Autodesk Inventor part; units mm, degrees
ref_plane "Work Plane1" through (0, 0, -22) normal (0, 0, -1) x (-1, 0, 0)
ref_plane "YZ Plane" through (0, 0, 0) normal (1, 0, 0) x (0, 1, 0)
ref_plane "XZ Plane" through (0, 0, 0) normal (0, 1, 0) x (-1, 0, 0)
sketch "Sketch1" plane through (0, 0, 0) normal (0, 0, 1) x (1, 0, 0)
  line L0 (-2.3383, -4.05) -> (-4.6765, 0)
  line L1 (-4.6765, 0) -> (-2.3383, 4.05)
  line L2 (-2.3383, 4.05) -> (2.3383, 4.05)
  line L3 (2.3383, 4.05) -> (4.6765, 0)
  line L4 (4.6765, 0) -> (2.3383, -4.05)
  line L5 (2.3383, -4.05) -> (-2.3383, -4.05)
  point P0 (0, 0)
  point P1 (0, 0)
  dimension "d0" = 4.05
extrude "Extrusion1" add sketch "Sketch1" against normal blind 44
sketch "Sketch2" plane through (4.6765, 0, 0) normal (0.866, 0.5, 0) x (0, 0, -1)
  line L0 (0, 4.6765) -> (0, 0)
  line L1 (4.75, 5.1383) -> (7.25, 5.1383)
  line L2 (7.25, 5.1383) -> (7.25, -0.4617)
  line L3 (7.25, -0.4617) -> (4.75, -0.4617)
  line L4 (4.75, -0.4617) -> (4.75, 5.1383)
  line L5 (4.75, 5.1383) -> (7.25, -0.4617) construction
  line L6 (7.25, 5.1383) -> (4.75, -0.4617) construction
  point P0 (0, 2.3383)
  point P1 (6, 2.3383)
  dimension "d3" = 2.5
  dimension "d4" = 5.6
  dimension "d10" = 0
  dimension "d11" = 6
extrude "Extrusion2" [suppressed]
sketch "Sketch3" plane through (0, 0, 0) normal (0, 0, 1) x (1, 0, 0)
  circle A0 centre (0, 0) radius 1.5
  dimension "d7" = 3
extrude "Extrusion3" cut sketch "Sketch3" against normal blind 8
ref_plane "Work Plane1" through (0, 0, -22) normal (0, 0, -1) x (-1, 0, 0)
mirror "Mirror1" [suppressed]
sketch "Sketch4" plane through (1.5014, 4.1, -7.25) normal (0, 0, 1) x (1, 0, 0)
  line L0 (0, 0) -> (-4.5469, -2.6251)
  line L1 (-1.7469, -7.4749) -> (-4.5469, -2.6251)
  line L2 (2.8, -4.8497) -> (-1.7469, -7.4749)
  line L3 (-4.5469, -2.6251) -> (-4.5469, -5.8583)
  line L4 (-1.7469, -7.4749) -> (-4.5469, -5.8583)
  line L5 (-1.7469, -7.4749) -> (-4.5469, -2.6251)
  point P0 (-1.5014, -4.1)
  dimension "d12" = 120
  dimension "d13" = 120
extrude "Extrusion4" [suppressed]
sketch "Sketch5" plane through (-4.6765, 0, -44) normal (-0.866, -0.5, 0) x (0, 0, 1)
  line L0 (0, -4.6765) -> (0, 0)
  line L1 (4.75, 0.5197) -> (7.25, 0.5197)
  line L2 (7.25, 0.5197) -> (7.25, -5.0803)
  line L3 (7.25, -5.0803) -> (4.75, -5.0803)
  line L4 (4.75, -5.0803) -> (4.75, 0.5197)
  line L5 (4.75, 0.5197) -> (7.25, -5.0803) construction
  line L6 (7.25, 0.5197) -> (4.75, -5.0803) construction
  line L7 (0, -3.8671) -> (0, -0.8671)
  line L8 (0, -4.6765) -> (0, 0)
  line L9 (0, 0) -> (0, 2.3383)
  line L10 (0, 2.3383) -> (0, 0)
  line L11 (0, 0) -> (0, -4.6765)
  line L12 (0, -4.6765) -> (0, -7.0148)
  line L13 (0, -7.0148) -> (0, -4.6765)
  line L14 (9.5, -0.8671) -> (9.5, -3.8671)
  line L15 (0, -3.8671) -> (0, -0.8671)
  line L16 (44, -7.0148) -> (0, -7.0148)
  line L17 (44, 2.3383) -> (0, 2.3383)
  point P0 (44, -2.3383)
  point P1 (6, -2.2803)
  dimension "d16" = 2.5
  dimension "d17" = 5.6
  dimension "d18" = 6
  dimension "d25" = 1.9345
extrude "Extrusion5" [suppressed]
sketch "Sketch6" plane through (-1.5019, -4.1, -42.75) normal (0, 0, -1) x (-1, 0, 0)
  line L0 (-1.7472, 7.4751) -> (-4.5472, 2.6253)
  line L1 (-4.5472, 2.6253) -> (-4.5472, 5.8585)
  line L2 (-1.7472, 7.4751) -> (-4.5472, 5.8585)
  line L3 (2.7993, 4.8501) -> (-1.7472, 7.4751)
  line L4 (0, 0) -> (-4.5472, 2.6253)
  line L5 (-1.7472, 7.4751) -> (-4.5472, 2.6253)
  point P0 (-1.5019, 4.1)
  dimension "d21" = 120
  dimension "d22" = 120
extrude "Extrusion6" [suppressed]
sketch "Sketch8" plane through (0, 0, -44) normal (0, 0, -1) x (-1, 0, 0)
  line L0 (-2.8, 1.25) -> (2.8, 1.25)
  line L1 (2.8, 1.25) -> (2.8, -1.25)
  line L2 (2.8, -1.25) -> (-2.8, -1.25)
  line L3 (-2.8, -1.25) -> (-2.8, 1.25)
  circle A0 centre (0, 0) radius 1.5
  line L4 (-2.8, 1.25) -> (2.8, -1.25) construction
  line L5 (2.8, 1.25) -> (-2.8, -1.25) construction
  dimension "d32" = 5.6
  dimension "d33" = 2.5
extrude "Extrusion8" cut sketch "Sketch8" against normal blind 6.5 contours L0 A0 L2 L3 | L0 A0 L2 | L0 L1 L2 A0
sketch "Sketch9" plane through (-2.3383, 4.05, 0) normal (0, 1, 0) x (1, 0, 0)
  line L0 (4.6765, 0) -> (4.6765, 44)
  line L1 (0, 44) -> (4.6765, 44)
  line L2 (0, 0) -> (0, 44)
  line L3 (0, 0) -> (4.6765, 0)
  line L4 (5.1383, 44) -> (-0.4617, 44)
  line L5 (2.3383, 44) -> (2.3383, 0) construction
  line L6 (2.3383, 44) -> (46.3383, 44) construction
  circle A0 centre (2.3383, 39.5) radius 1.5
  dimension "d36" = 90
  dimension "d37" = 3
  dimension "d38" = 0
  dimension "d39" = 4.5
extrude "Extrusion9" cut sketch "Sketch9" against normal up to surface (8.1 mm away) contours A0
sketch "Sketch10" plane through (-2.8, 1.25, -44) normal (0, -1, 0) x (1, 0, 0)
  circle A0 centre (2.8, 4.5) radius 1.5
  line L0 (5.6, 0) -> (0, 0)
  line L1 (5.6, 0) -> (5.6, 6.5)
  line L2 (5.6, 6.5) -> (0, 6.5)
  line L3 (0, 0) -> (0, 6.5)
  line L4 (0, 6.5) -> (2.8, 8.1166)
  line L5 (0, 6.5) -> (3.9156, 6.5) construction
  line L6 (5.6, 6.5) -> (2.8, 8.1166)
  line L7 (5.6, 6.5) -> (8.8332, 6.5) construction
  line L8 (5.6, 6.5) -> (0, 6.5)
  point P0 (2.8, 44)
  dimension "d42" = 30
  dimension "d43" = 150
extrude "Extrusion10" cut sketch "Sketch10" along normal blind 2.5 contours L2 L4 L6
sketch "Sketch11" plane through (-2.3383, 4.05, 0) normal (0, 1, 0) x (1, 0, 0)
  circle A0 centre (2.3383, 39.5) radius 1.5
  line L0 (0, 0) -> (4.6765, 0)
  line L1 (4.6765, 0) -> (4.6765, 44)
  line L2 (0, 44) -> (4.6765, 44)
  line L3 (0, 0) -> (0, 44)
  line L4 (-0.4617, 0.8) -> (5.1383, 0.8)
  line L5 (5.1383, 0.8) -> (5.1383, 3.3)
  line L6 (5.1383, 3.3) -> (-0.4617, 3.3)
  line L7 (-0.4617, 3.3) -> (-0.4617, 0.8)
  line L8 (-0.4617, 0.8) -> (5.1383, 3.3) construction
  line L9 (5.1383, 0.8) -> (-0.4617, 3.3) construction
  point P0 (2.3383, 0)
  point P1 (2.3383, 2.05)
  dimension "d46" = 5.6
  dimension "d47" = 2.5
  dimension "d48" = 2.05
extrude "Extrusion11" cut sketch "Sketch11" against normal blind 5.85 contours L4 L7 L6 L3 | L3 L6 L1 L4 | L1 L6 L5 L4
sketch "Sketch12" plane through (2.3383, 4.05, -0.8) normal (0, 0, -1) x (-1, 0, 0)
  line L0 (5.1383, -0.7997) -> (4.6765, 0)
  line L1 (5.1383, -0.7997) -> (5.1383, -5.85)
  line L2 (5.1383, -5.85) -> (-0.4617, -5.85)
  line L3 (-0.4617, -0.7997) -> (-0.4617, -5.85)
  line L4 (0, 0) -> (-0.4617, -0.7997)
  line L5 (4.6765, 0) -> (0, 0)
  circle A0 centre (2.3383, -4.05) radius 1.5
  line L6 (5.1383, -5.85) -> (2.3383, -7.4666)
  line L7 (5.1383, -5.85) -> (8.4476, -5.85) construction
  line L8 (-0.4617, -5.85) -> (2.3383, -7.4666)
  line L9 (-0.4617, -5.85) -> (2.7714, -5.85) construction
  dimension "d52" = 150
  dimension "d53" = 30
extrude "Extrusion12" cut sketch "Sketch12" along normal up to surface (2.5 mm away) contours L6 L8 L2
properties part number "SupportSecondToCoverNew" material "ABS Plastic"
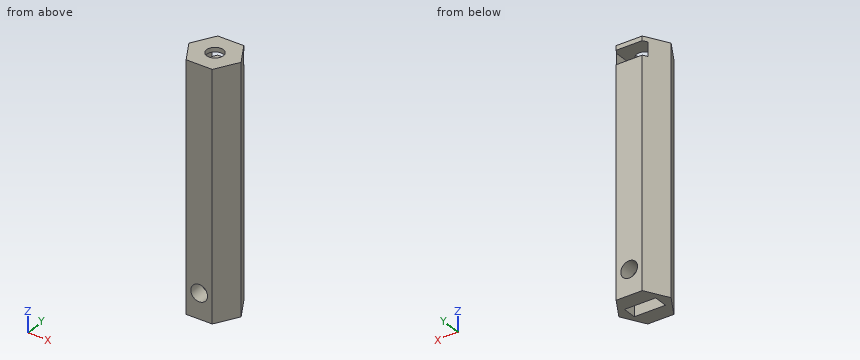
Part model, mm, in its own coordinate system. Round coordinates to 2 decimals unless told otherwise and drop trailing zeros. Loops run counter-clockwise (first coordinate to the right, second up) from the corner with the lowest first, then second, coordinate; pieces in that order, holes last. Notation, with made-up numbers: (9.5, 52) -> (32.5, 52) arc R20 ccw to (32.5, 61) -> close; hole circle Ø11 at (-6.75, -27.75). An arc over 180 degrees is marked (long way). Use CSV: the item, a comma, the result in double quotes. Start each with the question number.
1) Cut at D-D, the plane z = -16. Write the cut outline in (x, y), plus the area to 3 significant figures.
2) Cut at A-A, the plane z = -39.5. Write the cut outline in (x, y).
3) Drop flat-ended pins along their axis: P1, Ø3.5, axis at x = 0, y = 0, coming from the +Z side; P2, Ø2, axis at y = -0.5, z = -42, coming from the +X side; P3, Ø1.2, axis at y = 1.5, z = -2.5, coming from the -X side; P4, Ø1.5, axis at x = 0.5, y = -0.5, coming from the +Z side. Give the stop position or say it passes through.
4) Cut at C-C, the plane x = -0.5. Write the cut outline in (y, z).
5) Wall check: L1, parallel to Z at x = 0, y = -3.15; L2, parallel to Z at x = -0.75, y = -2; L3, parallel to Z at x = 2, y = -2. Give the ranges that are in metal, low to high. Write a range as [from, to].
6) Cut at B-B, the plane z = -6. Write the cut outline in (x, y).
Determined:
1,outline,"(-4.68, 0) -> (-2.34, -4.05) -> (2.34, -4.05) -> (4.68, 0) -> (2.34, 4.05) -> (-2.34, 4.05) -> close"
1,area,"56.8 mm2"
2,outline,"(-4.68, 0) -> (-2.34, -4.05) -> (-1.5, -4.05) -> (-1.5, -1.25) -> (-2.8, -1.25) -> (-2.8, 1.25) -> (-1.5, 1.25) -> (-1.5, 4.05) -> (-2.34, 4.05) -> close; (1.5, -4.05) -> (2.34, -4.05) -> (4.68, 0) -> (2.34, 4.05) -> (1.5, 4.05) -> (1.5, 1.25) -> (2.8, 1.25) -> (2.8, -1.25) -> (1.5, -1.25) -> close"
3,P1,"stops at z = 0"
3,P2,"stops at x = 4.68"
3,P3,"stops at x = -4.16"
3,P4,"stops at z = -8"
4,outline,"(-4.05, -44) -> (-1.25, -44) -> (-1.25, -40.91) -> (-4.05, -40.91) -> close; (-4.05, -38.09) -> (-1.25, -38.09) -> (-1.25, -36.17) -> (1.25, -36.17) -> (1.25, -38.09) -> (4.05, -38.09) -> (4.05, -3.3) -> (1.41, -3.3) -> (1.41, -8) -> (-1.41, -8) -> (-1.41, -3.3) -> (-3.13, -3.3) -> (-3.13, -0.8) -> (-1.41, -0.8) -> (-1.41, 0) -> (-4.05, 0) -> close; (1.25, -44) -> (4.05, -44) -> (4.05, -40.91) -> (1.25, -40.91) -> close; (1.41, -0.8) -> (4.05, -0.8) -> (4.05, 0) -> (1.41, 0) -> close"
5,L1,"z = [-44, -41], [-38, -3.3], [-0.8, 0]"
5,L2,"z = [-44, -40.8], [-38.2, -3.3], [-0.8, 0]"
5,L3,"z = [-44, -3.3], [-0.8, 0]"
6,outline,"(-4.68, 0) -> (-2.34, -4.05) -> (2.34, -4.05) -> (4.68, 0) -> (2.34, 4.05) -> (-2.34, 4.05) -> close; hole circle Ø3 at (0, 0)"
